Could you check a few things on this model? Use its own coordinates, in mm. A direction names the side the tool comes from. Give positions to 0.01 mm unless a question says otherwise; leave off trailing zeros. Loops run counter-clockwise (first coordinate to the right, second up) from the corner with the lowest first, then second, coordinate; pieces in that order, holes last. Notation, with made-up numbers: (67.25, -31) -> (107.25, -31) arc R19 cw to (107.25, -7) -> close; hole circle Ø3 at (13, -20.5). An arc over 180 degrees is marked (long way). Put each result on its own line as item: value.
```python
from build123d import *

# Parameters (mm, degrees)
SKETCH1_R           = 1.5
BOSS_EXTRUDE1_DEPTH = 2
SKETCH2_R           = 1.5
BOSS_EXTRUDE2_DEPTH = 6


with BuildPart() as part:
    # Sketch1 → Boss-Extrude1 (new body)
    with BuildSketch(Plane.XY):
        with BuildLine():
            Line((0, 4), (30, 4))
            ThreePointArc((30, 4), (34, 0), (30, -4))
            Line((30, -4), (0, -4))
            ThreePointArc((0, -4), (-4, 0), (0, 4))
        make_face()
        Circle(SKETCH1_R, mode=Mode.SUBTRACT)
    extrude(amount=BOSS_EXTRUDE1_DEPTH)

    # Sketch2 → Boss-Extrude2 (add)
    with BuildSketch(Plane.XY.offset(2)):
        with Locations((30, 0)):
            Circle(SKETCH2_R)
    extrude(amount=BOSS_EXTRUDE2_DEPTH)


solid = part.part
```
1. I need wall thicknesses on line 1 (Y direction, x = 0, z = 1.3); line 2 (Z direction, x = 8.5, y = -3.5); line 3 (X direction, y = 0.25, z = 1.5). Which ranges of each line are inside material? Lowest first, please.
Recorded:
line 1: y = -4 to -1.5, 1.5 to 4
line 2: z = 0 to 2
line 3: x = -3.99 to -1.48, 1.48 to 33.99
2. If we section it at D-D (x = 10): List the corners of the cut face in (y, z) for me, then the cut area to 3 significant figures.
Recorded:
outline: (-4, 0) -> (4, 0) -> (4, 2) -> (-4, 2) -> close
area: 16.0 mm^2
3. If we section it at C-C (z = 6.75): List the corners of the cut face in (x, y) for me, then the cut area to 3 significant figures.
Recorded:
outline: circle Ø3 at (30, 0)
area: 7.07 mm^2
4. I'm going to push a flat-ended pin straight in: pin 1 (4 mm diameter, centred on x = 8.5, y = 0, fed in from +Z). Where does the tip first touch, or does it pass through?
Recorded:
pin 1: stops at z = 2
5. If we section it at B-B (z = 0.75): List the corners of the cut face in (x, y) for me.
Recorded:
outline: (0, -4) -> (30, -4) arc R4 ccw to (30, 4) -> (0, 4) arc R4 ccw to start; hole circle Ø3 at (0, 0)
6. For faces 5 (the face through (15, 4, 1)), 6 (the face through (28.5, 0.07, 4.96)), which set-ups out of +Z, -Z, +X, -X, +Y, -Y let a thin tool reach every point of the face, with its end or its side?
Recorded:
face 5: +Z, -Z, +X, -X, +Y
face 6: +Z
7. Thinking about a two-plate mould opening in X: for faces 1 (the face through (-4, 0, 1)), 2 (the face through (-1.5, 0.07, 0.99)), 3 (the face through (34, 0, 1)), 4 (the face through (30, 0, 8)), which applies, pulls with the +X half, pulls with the -X half, needs draft (parallel to the pull), parting line crosses it, or undercut?
Recorded:
face 1: pulls with the -X half
face 2: undercut
face 3: pulls with the +X half
face 4: needs draft
8. If we section it at A-A (y = 0): List the corners of the cut face in (x, z) for me, then the cut area to 3 significant figures.
Recorded:
outline: (-4, 0) -> (-1.5, 0) -> (-1.5, 2) -> (-4, 2) -> close; (1.5, 0) -> (34, 0) -> (34, 2) -> (31.5, 2) -> (31.5, 8) -> (28.5, 8) -> (28.5, 2) -> (1.5, 2) -> close
area: 88.0 mm^2
